Part print with two shaded views. Sizes in mm from the minimum x, y, z corner. A direction names the side the tool comes from. Coordinates: 2 decimals unless noted, no trailing zeros. Write each loop counter-clockwise with the first axis right and the second up, starting at its lowest first coordinate (ties: lowest second). Pieces come first, ordered by that corner, then holes. Notation, with made-up numbers: (-12.75, -31.75) - (33.25, -31.75) arc R17 cw to (33.25, -27.75) - close; hole circle Ø1 at (-7, -38). An arc over 180 degrees is marked (long way). Answer in a Markdown table with one row per item. Add a question column.
Q1. Pin check, flat tip, straight feed: pin 1 (8.5 mm diameter, centred on x = 134.76, z = 24.76, fed in from +Y). Stop position of the tip, or through.
Q2. Drill centre lines: line 1 along Z through (x, y) = (26.5, 8.5); line 2 along X through (y, z) = (17.5, 22); line 3 along Y through (x, z) = (140.5, 80.5). Where is each one in solid material? Low to high. Write a range as from..to.
Q3. Two-plate mould, pull along X, no slides. Class the marked faces 1, 2, 3 and 4: +X half, -X half, draft (parallel to the pull), parting line (faces both ways), or undercut.
Q4. Band-saw the part on B-B (y = 11.5). List the corners of the cut face in (x, z).
Q5. 3-axis set-ups, long thin cutter, end or side, ignore diameter. For the marked faces 5 and 6: which of +Z, -Z, +X, -X, +Y, -Y reach the whole face in a straight line?
Q6. Band-saw the part on A-A (x = 124.5). List the corners of the cut face in (y, z), and give its area (3 significant figures).
Q7. Band-saw the part on C-C (z = 44). List the corners of the cut face in (x, y).
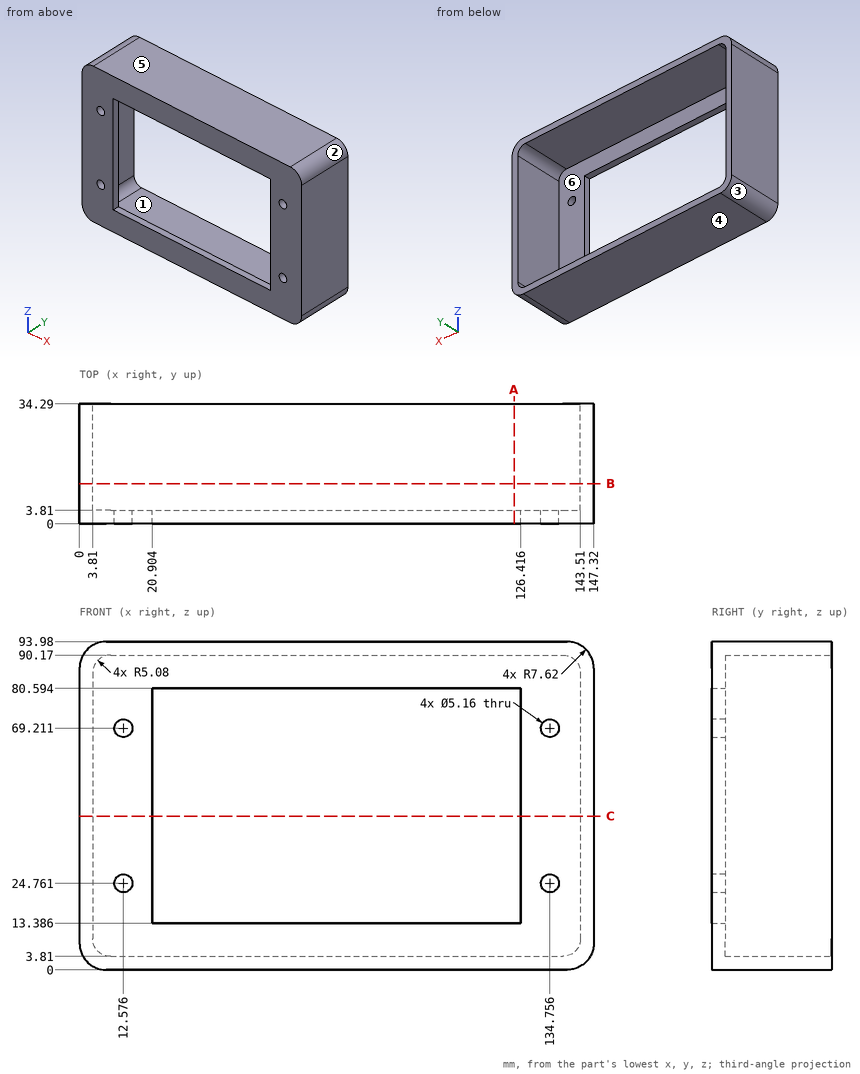
Checked values:
| question | item | result |
|---|---|---|
| 1 | pin 1 | stops at y = 3.81 |
| 2 | line 1 | z = 0..3.81, 90.17..93.98 |
| 2 | line 2 | x = 0..3.81, 143.51..147.32 |
| 2 | line 3 | y = 0..3.81 |
| 3 | face 1 | undercut |
| 3 | face 2 | +X half |
| 3 | face 3 | -X half |
| 3 | face 4 | draft |
| 4 | outline | (0, 7.62) arc R7.62 ccw to (7.62, 0) - (139.7, 0) arc R7.62 ccw to (147.32, 7.62) - (147.32, 86.36) arc R7.62 ccw to (139.7, 93.98) - (7.62, 93.98) arc R7.62 ccw to (0, 86.36) - close; hole (3.81, 8.89) arc R5.08 ccw to (8.89, 3.81) - (138.43, 3.81) arc R5.08 ccw to (143.51, 8.89) - (143.51, 85.09) arc R5.08 ccw to (138.43, 90.17) - (8.89, 90.17) arc R5.08 ccw to (3.81, 85.09) - close |
| 5 | face 5 | +Z, +X, -X, +Y, -Y |
| 5 | face 6 | +Y |
| 6 | outline | (0, 0) - (34.29, 0) - (34.29, 3.81) - (3.81, 3.81) - (3.81, 13.39) - (0, 13.39) - close; (0, 80.59) - (3.81, 80.59) - (3.81, 90.17) - (34.29, 90.17) - (34.29, 93.98) - (0, 93.98) - close |
| 6 | area | 334 mm² |
| 7 | outline | (0, 0) - (20.9, 0) - (20.9, 3.81) - (3.81, 3.81) - (3.81, 34.29) - (0, 34.29) - close; (126.42, 0) - (147.32, 0) - (147.32, 34.29) - (143.51, 34.29) - (143.51, 3.81) - (126.42, 3.81) - close |
